from build123d import *

# Parameters (mm, degrees)
SKETCH_1_R      = 300
EXTRUDE_1_DEPTH = 50
SKETCH_2_W      = 500
SKETCH_2_H      = 500
EXTRUDE_2_DEPTH = 50
SKETCH_3_W      = 500
SKETCH_3_H      = 50
EXTRUDE_3_DEPTH = 600


with BuildPart() as part:
    # 草图1 → 凸台-拉伸1 (new body)
    with BuildSketch(Plane.XY):
        Circle(SKETCH_1_R)
    extrude(amount=EXTRUDE_1_DEPTH)

    # 草图2 → 凸台-拉伸2 (add)
    with BuildSketch(Plane.XY):
        Rectangle(SKETCH_2_W, SKETCH_2_H)
    extrude(amount=EXTRUDE_2_DEPTH)

    # 草图3 → 凸台-拉伸3 (add)
    with BuildSketch(Plane.XY):
        with Locations((0, 225)):
            Rectangle(SKETCH_3_W, SKETCH_3_H)
    extrude(amount=EXTRUDE_3_DEPTH)


solid = part.part
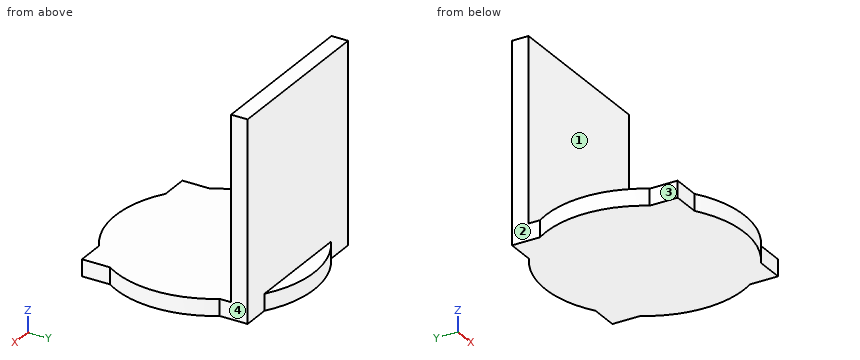
Design review of the part built by this model. Coordinates are the model's own, in mm. Face numbers are marked on the shaded views. A direction names the side the tool comes from. Give positions to 0.01 mm unless a question says otherwise; leave off trailing zeros. Loops run counter-clockwise (first coordinate to the right, second up) from the corner with the lowest first, then second, coordinate; pieces in that order, holes last. Notation, with made-up numbers: M 22.5,88 L 47.5,88 A27 cw 47.5,127 Z; hole C -30.75,-18.75 d7. An arc over 180 degrees is marked long. Answer as a JSON object with one key per item and string values.
Item 1: We need section B-B (z = 41). State the section outline as (x, y) points.
Output values:
{"outline": "M -250,-250 L -165.83,-250 A300 ccw 165.83,-250 L 250,-250 L 250,-165.83 A300 ccw 250,165.83 L 250,250 L 165.83,250 A300 ccw -165.83,250 L -250,250 L -250,165.83 A300 ccw -250,-165.83 Z"}
Item 2: Machinability: for the marked faces 1, 2, 3 and 4, which of the approach directions +Z, -Z, +X, -X, +Y, -Y give a long, thin tool a straight path to every point of the face, cutting with its end or side? Answer none if there is none.
Output values:
{"face 1": "+Z, +X, -X, -Y", "face 2": "+Z, -Z, -X, +Y", "face 3": "+Z, -Z, -X, -Y", "face 4": "+Z, -Z, +X, +Y"}
Item 3: Wall thickness on line 1 along Z through (x, y) = (-40, 251); line 2 along Y through (x, z) = (179.5, 242.5); line 3 along X through (y, z) = (244, 466.5): over which ranges is each line inside the solid? List them lowest first.
Output values:
{"line 1": "z = 0 to 50", "line 2": "y = 200 to 250", "line 3": "x = -250 to 250"}
Item 4: We need section C-C (y = 84). State the section outline as (x, z) points, and give its area (3 significant figures).
Output values:
{"outline": "M -288,0 L 288,0 L 288,50 L -288,50 Z", "area": "28,800 mm2"}
Item 5: We need section D-D (x = -25). State the section outline as (y, z) points, and give its area (3 significant figures).
Output values:
{"outline": "M -298.96,0 L 298.96,0 L 298.96,50 L 250,50 L 250,600 L 200,600 L 200,50 L -298.96,50 Z", "area": "57,400 mm2"}
Item 6: For P1, Ø10, axis at x = 81.5, z = 526, coming from the +Y side; P2, Ø2, axis at x = 177, y = -214.5, coming from the +Z side; P3, Ø1, axis at x = -191, y = 44, coming from the -Z side; P4, Ø15, axis at y = -204.5, z = 29, coming from the +X side, all flat-tipped, find the tip position at first contact; note any pin that passes through.
Output values:
{"P1": "stops at y = 250", "P2": "stops at z = 50", "P3": "stops at z = 0", "P4": "stops at x = 250"}
Item 7: We need section A-A (x = -231.5). State the section outline as (y, z) points.
Output values:
{"outline": "M -250,0 L 250,0 L 250,600 L 200,600 L 200,50 L -250,50 Z"}
